Verification items for the finished model (mm, model axes). A direction names the side the tool comes from. Coordinates: 2 decimals unless noted, no trailing zeros. Write each loop counter-clockwise with the first axis right and the second up, starting at its lowest first coordinate (ties: lowest second). Pieces come first, ordered by that corner, then holes.
```python
from build123d import *

# Parameters (mm, degrees)
SKETCH_1_R             = 35
SKETCH_1_R_2           = 8
EXTRUDE_1_DEPTH        = 310
SKETCH_2_W             = 1600
SKETCH_2_H             = 290
CUT_EXTRUDE_1_DEPTH    = 913.931541793
SKETCH_3_R             = 100
SKETCH_3_R_2           = 6
SKETCH_3_R_3           = 42.5
CUT_EXTRUDE_2_DEPTH    = 10
EXTRUDE_2_DEPTH        = 330
SKETCH_6_W             = 300
SKETCH_6_H             = 260
EXTRUDE_3_DEPTH        = 10
SKETCH_7_W             = 300
SKETCH_7_H             = 260
EXTRUDE_4_DEPTH        = 10
SKETCH_9_W             = 10
SKETCH_9_H             = 290
EXTRUDE_5_DEPTH        = 184
SKETCH_10_W            = 420
SKETCH_10_H            = 290
EXTRUDE_6_DEPTH        = 6
SKETCH_11_R            = 85
SKETCH_11_R_2          = 42.5
SKETCH_11_R_3          = 8
EXTRUDE_7_DEPTH        = 10
SKETCH_12_R            = 85
SKETCH_12_R_2          = 35
SKETCH_12_R_3          = 8
EXTRUDE_8_DEPTH        = 10
PATTERN_LINEAR_2_COUNT = 2
PATTERN_LINEAR_2_PITCH = 800
SKETCH_13_R            = 150
SKETCH_13_R_2          = 100
SKETCH_13_R_3          = 6
EXTRUDE_9_DEPTH        = 24
SKETCH_14_R            = 115
CUT_EXTRUDE_3_DEPTH    = 6
SKETCH_17_W            = 344
SKETCH_17_H            = 330
EXTRUDE_11_DEPTH       = 20
SKETCH_16_W            = 320
SKETCH_16_H            = 330
EXTRUDE_10_DEPTH       = 5


with BuildPart() as part:
    # Sketch 1 → Extrude 1 (new body)
    with BuildSketch(Plane.XY):
        with BuildLine():
            Line((-740, 0), (740, 0))
            Line((740, 0), (800, 52))
            Line((800, 52), (800, 312))
            Line((800, 312), (400, 312))
            ThreePointArc((400, 312), (303.608851243, 286.659738783), (232.141956451, 217.191290218))
            ThreePointArc((232.141956451, 217.191290218), (211.645136257, 197.267627611), (184, 190))
            Line((184, 190), (-184, 190))
            ThreePointArc((-184, 190), (-211.645136257, 197.267627611), (-232.141956451, 217.191290218))
            ThreePointArc((-232.141956451, 217.191290218), (-303.608851243, 286.659738783), (-400, 312))
            Line((-400, 312), (-800, 312))
            Line((-800, 312), (-800, 52))
            Line((-800, 52), (-740, 0))
        make_face()
        with Locations((-400, 116)):
            Circle(SKETCH_1_R, mode=Mode.SUBTRACT)
        with Locations((400, 116)):
            Circle(SKETCH_1_R, mode=Mode.SUBTRACT)
        with Locations((-445, 66)):
            Circle(SKETCH_1_R_2, mode=Mode.SUBTRACT)
        with Locations((-355, 66)):
            Circle(SKETCH_1_R_2, mode=Mode.SUBTRACT)
        with Locations((355, 66)):
            Circle(SKETCH_1_R_2, mode=Mode.SUBTRACT)
        with Locations((445, 66)):
            Circle(SKETCH_1_R_2, mode=Mode.SUBTRACT)
    extrude(amount=EXTRUDE_1_DEPTH)

    # Sketch 2 → Cut-Extrude 1 (cut, through all)
    with BuildSketch(Plane(origin=(0, 0, 0), x_dir=(-1, 0, 0), z_dir=(0, -1, 0))):
        with Locations((0, -155)):
            Rectangle(SKETCH_2_W, SKETCH_2_H)
    extrude(amount=-CUT_EXTRUDE_1_DEPTH, mode=Mode.SUBTRACT)


with BuildPart() as cut_extrude_1_piece_1:
    # of the separate pieces the step leaves, piece 1, a body of its own (cut_extrude_1_pieces)
    add(part.part.solids().sort_by_distance((-740, 0, 0))[0])

    # Sketch 5 → Extrude 2 (add)
    with BuildSketch(Plane.XY.offset(-10)):
        with BuildLine():
            Line((485, 312), (485, 318))
            Line((485, 318), (400, 318))
            ThreePointArc((400, 318), (300.658101791, 291.8840165), (227.003444914, 220.288982775))
            ThreePointArc((227.003444914, 220.288982775), (208.694386805, 202.491905329), (184, 196))
            Line((184, 196), (-184, 196))
            ThreePointArc((-184, 196), (-208.694386805, 202.491905329), (-227.003444914, 220.288982775))
            ThreePointArc((-227.003444914, 220.288982775), (-300.658101791, 291.8840165), (-400, 318))
            Line((-400, 318), (-485, 318))
            Line((-485, 318), (-485, 312))
            Line((-485, 312), (-400, 312))
            ThreePointArc((-400, 312), (-303.608851243, 286.659738783), (-232.141956451, 217.191290218))
            ThreePointArc((-232.141956451, 217.191290218), (-211.645136257, 197.267627611), (-184, 190))
            Line((-184, 190), (184, 190))
            ThreePointArc((184, 190), (211.645136257, 197.267627611), (232.141956451, 217.191290218))
            ThreePointArc((232.141956451, 217.191290218), (303.608851243, 286.659738783), (400, 312))
            Line((400, 312), (485, 312))
        make_face()
    extrude(amount=EXTRUDE_2_DEPTH)



with BuildPart() as cut_extrude_1_piece_2:
    # of the separate pieces the step leaves, piece 2, a body of its own (cut_extrude_1_pieces)
    add(part.part.solids().sort_by_distance((-740, 0, 300))[0])

    # Sketch 3 → Cut-Extrude 2 (cut)
    with BuildSketch(Plane.XY.offset(310)):
        with Locations((-641.476706951, 151)):
            Circle(SKETCH_3_R)
        with Locations((641.476706951, 151)):
            Circle(SKETCH_3_R)
        with Locations((-735.168355458, 244.691648507)):
            Circle(SKETCH_3_R_2)
        with Locations((-547.785058444, 244.691648507)):
            Circle(SKETCH_3_R_2)
        with Locations((-735.168355458, 57.308351493)):
            Circle(SKETCH_3_R_2)
        with Locations((-547.785058444, 57.308351493)):
            Circle(SKETCH_3_R_2)
        with Locations((547.785058444, 244.691648507)):
            Circle(SKETCH_3_R_2)
        with Locations((735.168355458, 244.691648507)):
            Circle(SKETCH_3_R_2)
        with Locations((735.168355458, 57.308351493)):
            Circle(SKETCH_3_R_2)
        with Locations((547.785058444, 57.308351493)):
            Circle(SKETCH_3_R_2)
        with Locations((-400, 116)):
            Circle(SKETCH_3_R_3)
        with Locations((400, 116)):
            Circle(SKETCH_3_R_3)
    extrude(amount=-CUT_EXTRUDE_2_DEPTH, mode=Mode.SUBTRACT)


with BuildPart() as cut_extrude_1_piece_1_1:
    add(cut_extrude_1_piece_1.part)

    add(cut_extrude_1_piece_2.part)  # Extrude 3 merges Cut-Extrude 1 piece 2
    # Sketch 6 → Extrude 3 (add)
    with BuildSketch(Plane(origin=(800, 0, 0), x_dir=(0, 0, -1), z_dir=(1, 0, 0))):
        with Locations((-155, 182)):
            Rectangle(SKETCH_6_W, SKETCH_6_H)
    extrude(amount=EXTRUDE_3_DEPTH)

    # Sketch 7 → Extrude 4 (add)
    with BuildSketch(Plane.ZY.offset(800)):
        with Locations((155, 182)):
            Rectangle(SKETCH_7_W, SKETCH_7_H)
    extrude(amount=EXTRUDE_4_DEPTH)

    # Sketch 9 → Extrude 5 (add)
    with BuildSketch(Plane.XZ.offset(-190)):
        with Locations((-105, 155)):
            Rectangle(SKETCH_9_W, SKETCH_9_H)
        with Locations((105, 155)):
            Rectangle(SKETCH_9_W, SKETCH_9_H)
        with Locations((155, 155)):
            Rectangle(SKETCH_9_W, SKETCH_9_H)
        with Locations((-155, 155)):
            Rectangle(SKETCH_9_W, SKETCH_9_H)
    extrude(amount=EXTRUDE_5_DEPTH)

    # Sketch 10 → Extrude 6 (add)
    with BuildSketch(Plane.XZ.offset(-6)):
        with Locations((0, 155)):
            Rectangle(SKETCH_10_W, SKETCH_10_H)
    extrude(amount=EXTRUDE_6_DEPTH)

    # Sketch 11 → Extrude 7 (add)
    with BuildSketch(Plane.XY.offset(310)):
        with Locations(Location((-400, 116, 0), (0, 0, 180))):
            Circle(SKETCH_11_R)
        with Locations((-400, 116)):
            Circle(SKETCH_11_R_2, mode=Mode.SUBTRACT)
        with Locations((-445, 66)):
            Circle(SKETCH_11_R_3, mode=Mode.SUBTRACT)
        with Locations((-355, 66)):
            Circle(SKETCH_11_R_3, mode=Mode.SUBTRACT)
    extrude_7 = extrude(amount=EXTRUDE_7_DEPTH)

    # Sketch 12 → Extrude 8 (add)
    with BuildSketch(Plane(origin=(0, 0, 0), x_dir=(-1, 0, 0), z_dir=(0, 0, -1))):
        with Locations((400, 116)):
            Circle(SKETCH_12_R)
        with Locations((400, 116)):
            Circle(SKETCH_12_R_2, mode=Mode.SUBTRACT)
        with Locations(Location((355, 66, 0), (0, 0, 180))):
            Circle(SKETCH_12_R_3, mode=Mode.SUBTRACT)
        with Locations(Location((445, 66, 0), (0, 0, 180))):
            Circle(SKETCH_12_R_3, mode=Mode.SUBTRACT)
    extrude_8 = extrude(amount=EXTRUDE_8_DEPTH)

    # Pattern Linear 2: Extrude 7, Extrude 8 ×2
    with Locations(*[(i * PATTERN_LINEAR_2_PITCH, 0, 0) for i in range(1, PATTERN_LINEAR_2_COUNT)]):
        add(extrude_7)
        add(extrude_8)

    # Sketch 13 → Extrude 9 (add)
    # profile 1 of 2: a face of its own
    with BuildSketch(Plane.XY.offset(310)):
        with Locations(Location((-641.476706951, 151, 0), (0, 0, 180))):
            Circle(SKETCH_13_R)
        with Locations((-641.476706951, 151)):
            Circle(SKETCH_13_R_2, mode=Mode.SUBTRACT)
        with Locations((-735.168355458, 244.691648507)):
            Circle(SKETCH_13_R_3, mode=Mode.SUBTRACT)
        with Locations((-547.785058444, 244.691648507)):
            Circle(SKETCH_13_R_3, mode=Mode.SUBTRACT)
        with Locations((-547.785058444, 57.308351493)):
            Circle(SKETCH_13_R_3, mode=Mode.SUBTRACT)
        with Locations((-735.168355458, 57.308351493)):
            Circle(SKETCH_13_R_3, mode=Mode.SUBTRACT)
    # profile 2 of 2: a face of its own
    with BuildSketch(Plane.XY.offset(310)):
        with Locations(Location((641.476706951, 151, 0), (0, 0, 180))):
            Circle(SKETCH_13_R)
        with Locations((735.168355458, 244.691648507)):
            Circle(SKETCH_13_R_3, mode=Mode.SUBTRACT)
        with Locations((547.785058444, 57.308351493)):
            Circle(SKETCH_13_R_3, mode=Mode.SUBTRACT)
        with Locations((735.168355458, 57.308351493)):
            Circle(SKETCH_13_R_3, mode=Mode.SUBTRACT)
        with Locations((547.785058444, 244.691648507)):
            Circle(SKETCH_13_R_3, mode=Mode.SUBTRACT)
        with Locations((641.476706951, 151)):
            Circle(SKETCH_13_R_2, mode=Mode.SUBTRACT)
    extrude(amount=EXTRUDE_9_DEPTH)

    # Sketch 14 → Cut-Extrude 3 (cut)
    with BuildSketch(Plane.XY.offset(334)):
        with Locations((-641.476706951, 151)):
            Circle(SKETCH_14_R)
        with Locations((641.476706951, 151)):
            Circle(SKETCH_14_R)
    extrude(amount=-CUT_EXTRUDE_3_DEPTH, mode=Mode.SUBTRACT)

    # Sketch 17 → Extrude 11 (add)
    with BuildSketch(Plane(origin=(0, 196, 0), x_dir=(1, 0, 0), z_dir=(0, 1, 0))):
        with Locations((0, -155)):
            Rectangle(SKETCH_17_W, SKETCH_17_H)
    extrude(amount=EXTRUDE_11_DEPTH)

    # Sketch 16 → Extrude 10 (add)
    with BuildSketch(Plane(origin=(0, 216, 0), x_dir=(1, 0, 0), z_dir=(0, 1, 0))):
        with Locations((0, -155)):
            Rectangle(SKETCH_16_W, SKETCH_16_H)
    extrude(amount=EXTRUDE_10_DEPTH)


solid = cut_extrude_1_piece_1_1.part
```
1. Draft check along X on faces 4 (the cylindrical face through (-549.1, 112.7, 313.8)), 5 (the flat face through (606.9, 245.2, 328)), 6 (the flat face through (185, 6, 157)). Enter one of: pulls with the +X half, pulls with the -X half, needs draft (parallel to the pull), parting line crosses it, or undercut.
2. Tool access check on faces 1 (the flat face through (800, 184, 157)), 2 (the cylindrical face through (-212, 197.47, 314.93)), 3 (the flat face through (-2, 221, 153)). Record the directions out of +Z, -Z, +X, -X, +Y, -Y that give a thin tool (end or side, any length) a straight path to the whole face; none if there is none.
3. Sectioned sample at B-B, the plane z = 177. Give the number of separate pieces and of enclosed holes in the cut face, and give its area (3 significant figures).
4. Sectioned sample at A-A, the plane x = 652. Record the boundary of the cut face in (y, z), and give its area (3 significant figures).
5. Material ranges on L1, parallel to X at y = 158, z = 245.5; L2, parallel to Z at x = -491, y = 215.5; L3, parallel to Y at x = -5.5, z = 114, recorded low to high.
6. Gauge pin test, flat ends, axial feed: P1, Ø15.5, axis at x = 547.79, y = 57.31, coming from the -Z side; P2, Ø8, axis at x = -395.5, z = 28, coming from the -Y side; P3, Ø4, axis at x = 389, z = 223.5, coming from the -Y side. Record the tip position at first contact, or that the pin passes through.
Outcome:
1. face 4: undercut
1. face 5: undercut
1. face 6: needs draft
2. face 1: +Y, -Y
2. face 2: +Z, -Y
2. face 3: +Z, -Z, +Y
3. separate pieces: 3
3. enclosed holes: 3
3. area: 29,900 mm2
4. outline: (0, 0) - (312, 0) - (312, 10) - (0, 10) - close; (0, 300) - (51.56, 300) - (51.56, 328) - (36.48, 328) - (36.48, 334) - (1.37, 334) - (1.37, 310) - (0, 310) - close; (250.44, 300) - (312, 300) - (312, 310) - (300.63, 310) - (300.63, 334) - (265.52, 334) - (265.52, 328) - (250.44, 328) - close
4. area: 6,480 mm2
5. L1: x = -810 to -800, -160 to -150, -110 to -100, 100 to 110, 150 to 160, 800 to 810
5. L2: z = 0 to 10, 300 to 310
5. L3: y = 0 to 6, 190 to 221
6. P1: stops at z = 0
6. P2: stops at y = 311.82
6. P3: stops at y = 311.57
